Can you work these out from the model? Positions are in its coordinate system, mm. A direction names the side the tool comes from. Round coordinates to 2 decimals unless told otherwise and drop trailing zeros. Loops run counter-clockwise (first coordinate to the right, second up) from the corner with the lowest first, then second, coordinate; pieces in that order, holes last. Notation, with made-up numbers: M 14.25,-35.75 L 63.25,-35.75 A24 cw 63.25,3.25 Z; hole C 64.25,42 d2. An arc over 180 degrees is marked long. Use a Markdown table: item, result. Add a question column.
```python
from build123d import *

# Parameters (mm, degrees)
SKETCH1_W           = 25.4
SKETCH1_H           = 64.6
BOSS_EXTRUDE1_DEPTH = 5
SKETCH2_R           = 1.35
SKETCH2_W           = 16.5
SKETCH2_H           = 3.5
CUT_EXTRUDE1_DEPTH  = 6
SKETCH3_R           = 1.75
CUT_EXTRUDE2_DEPTH  = 6


with BuildPart() as part:
    # Sketch1 → Boss-Extrude1 (new body)
    with BuildSketch(Plane.XY):
        with Locations((0, 122.3)):
            Rectangle(SKETCH1_W, SKETCH1_H)
    extrude(amount=-BOSS_EXTRUDE1_DEPTH)

    # Sketch2 → Cut-Extrude1 (cut, through all)
    with BuildSketch(Plane(origin=(0, 0, -5), x_dir=(-1, 0, 0), z_dir=(0, 0, -1))):
        with Locations((-10, 152.05)):
            Circle(SKETCH2_R)
        with Locations((10, 152.05)):
            Circle(SKETCH2_R)
        with Locations((-10, 139.55)):
            Circle(SKETCH2_R)
        with Locations((10, 139.55)):
            Circle(SKETCH2_R)
        with Locations((0, 139.55)):
            Rectangle(SKETCH2_W, SKETCH2_H)
    extrude(amount=-CUT_EXTRUDE1_DEPTH, mode=Mode.SUBTRACT)

    # Sketch3 → Cut-Extrude2 (cut, through all)
    with BuildSketch(Plane.XY):
        with Locations((-7.7, 94.48222968)):
            Circle(SKETCH3_R)
        with Locations((7.7, 94.48222968)):
            Circle(SKETCH3_R)
    extrude(amount=-CUT_EXTRUDE2_DEPTH, mode=Mode.SUBTRACT)


solid = part.part
```
(1) Suppose I cut it at A-A on y = 152.05. List the corners of the cut face in (x, z) for me, and give its area (3 significant figures).
(2) Suppose I cut it at B-B on x = 2.75. List the corners of the cut face in (y, z) for me, and give its area (4 significant figures).
(3) Suppose I cut it at D-D on z = -0.95. List the corners of the cut face in (x, y) for me, and give its area (3 significant figures).
(4) If I drill on probe 1 along X at (y, z) = (152.05, -1.75); probe 2 along Y at (x, z) = (-10, -2.05); probe 3 along X at (y, z) = (139.55, -1.8), over which ranges is the centre line in solid material (lowest first)? Write a range as [from, to].
(5) I'm going to push a flat-ended pin straight in: pin 1 (3 mm diameter, centred on x = 7.7, y = 94.48, fed in from +Z). Where does the tip first touch, or does it pass through?
(6) Thinking about a two-plate mould opening in X: for faces 3 (the face through (-8.25, 140, -3)), 4 (the face through (12.7, 122, -2)), 5 (the face through (0, 90, -2)), 6 (the face through (-12.7, 122, -2)), which applies, released by +X, released by -X, zero draft, split by the parting line, or undercut?
(7) On a 3-axis mill with a long thin cutter (end or side, diameter ignored), from which of +Z, -Z, +X, -X, +Y, -Y can I reach the whole of each face in a straight line? I mean faces 1 (the face through (0, 141.3, -3)), 2 (the face through (0, 123, -5)). Say none if no direction works.
(8) Suppose I cut it at C-C on x = -10.5. List the corners of the cut face in (y, z) for me, and give its area (3 significant figures).
Results below:
| question | item | result |
|---|---|---|
| 1 | outline | M -12.7,-5 L -11.35,-5 L -11.35,0 L -12.7,0 Z; M -8.65,-5 L 8.65,-5 L 8.65,0 L -8.65,0 Z; M 11.35,-5 L 12.7,-5 L 12.7,0 L 11.35,0 Z |
| 1 | area | 100 mm² |
| 2 | outline | M 90,-5 L 137.8,-5 L 137.8,0 L 90,0 Z; M 141.3,-5 L 154.6,-5 L 154.6,0 L 141.3,0 Z |
| 2 | area | 305.5 mm² |
| 3 | outline | M -12.7,90 L 12.7,90 L 12.7,154.6 L -12.7,154.6 Z; hole C -10,139.55 d2.7; hole C -10,152.05 d2.7; hole C -7.7,94.48 d3.5; hole M -8.25,137.8 L 8.25,137.8 L 8.25,141.3 L -8.25,141.3 Z; hole C 7.7,94.48 d3.5; hole C 10,139.55 d2.7; hole C 10,152.05 d2.7 |
| 3 | area | 1,540 mm² |
| 4 | probe 1 | x = [-12.7, -11.35], [-8.65, 8.65], [11.35, 12.7] |
| 4 | probe 2 | y = [90, 138.2], [140.9, 150.7], [153.4, 154.6] |
| 4 | probe 3 | x = [-12.7, -11.35], [-8.65, -8.25], [8.25, 8.65], [11.35, 12.7] |
| 5 | pin 1 | passes through |
| 6 | face 3 | undercut |
| 6 | face 4 | released by +X |
| 6 | face 5 | zero draft |
| 6 | face 6 | released by -X |
| 7 | face 1 | +Z, -Z |
| 7 | face 2 | -Z, +X, -X, +Y, -Y |
| 8 | outline | M 90,-5 L 138.3,-5 L 138.3,0 L 90,0 Z; M 140.8,-5 L 150.8,-5 L 150.8,0 L 140.8,0 Z; M 153.3,-5 L 154.6,-5 L 154.6,0 L 153.3,0 Z |
| 8 | area | 298 mm² |
